The listing builds one solid part. Answer for the finished solid, in the listing's coordinates (mm). Face numbers are marked on the shaded views. A direction names the side the tool comes from. Give positions to 0.01 mm unless a question says otherwise; leave off trailing zeros. Order: outer loops, then holes, each group sorted by start corner. A loop starts at its lowest first (then second) coordinate and runs counter-clockwise, first axis right, second up. Notation, with made-up numbers: (18.25, 68.5) - (56.25, 68.5) arc R20 ccw to (56.25, 99.5) - close; hole circle Ø1 at (-38.5, 11.25). An arc over 180 degrees is marked (long way). Answer in a Markdown table with one row per item.
from build123d import *

# Parameters (mm, degrees)
SKETCH1_W                   = 62.178178995
SKETCH1_H                   = 55.159619557
BOSS_EXTRUDE1_DEPTH         = 3.175
F_1_4_0_25_DIAMETER_HOLE1_D = 6.35
CUT_EXTRUDE6_DEPTH          = 84.179265432
FILLET1_R                   = 8.382
SKETCH7_W                   = 19.05
SKETCH7_H                   = 3.175
BOSS_EXTRUDE2_DEPTH         = 3.175


with BuildPart() as part:
    # Sketch1 → Boss-Extrude1 (new body)
    with BuildSketch(Plane.XY):
        with Locations((-31.089089498, 27.579809779)):
            Rectangle(SKETCH1_W, SKETCH1_H)
    extrude(amount=BOSS_EXTRUDE1_DEPTH)

    # 1/4 (0.25) Diameter Hole1 (through all)
    with Locations(Plane(origin=(0, 0, 0), x_dir=(-1, 0, 0), z_dir=(0, 0, -1))):
        with Locations((42.112178995, 18.542)):
            Hole(F_1_4_0_25_DIAMETER_HOLE1_D / 2)

    # Sketch4 → Cut-Extrude6 (cut, through all)
    with BuildSketch(Plane(origin=(0, 0, 0), x_dir=(-1, 0, 0), z_dir=(0, 0, -1))):
        Polygon((46.938178995, 26.4795), (62.178178995, 0), (62.178178995, 55.159619557), (0, 55.159619557), (0, 0), (24.636978995, 0), (36.778178995, 26.4795), align=None)
    extrude(amount=-CUT_EXTRUDE6_DEPTH, mode=Mode.SUBTRACT)

    # Fillet1
    # the kernel refuses this fillet: 8.382 mm, written as the material it takes off along each edge
    with BuildSketch(Plane(origin=(-46.938178995, 26.4795, -12.117368839), x_dir=(-0.49882253176769886, -0.8667041489463767, 0), z_dir=(0, 0, 1))) as fillet1_piece_1:
        with BuildLine():
            CenterArc((FILLET1_R * 0.578256685216, FILLET1_R), FILLET1_R, 209.922129856, 60.077870144)
            Line((-FILLET1_R * 0.288447463731, FILLET1_R * 0.501177468232), (0, 0))
            Line((0, 0), (FILLET1_R * 0.578256685216, 0))
        make_face()
    extrude(amount=27.409737677, mode=Mode.SUBTRACT)
    with BuildSketch(Plane(origin=(-36.778178995, 26.4795, -13.444588142), x_dir=(0.41678981361521655, -0.9090028884808855, 0), z_dir=(0, 0, 1))) as fillet1_piece_2:
        with BuildLine():
            CenterArc((FILLET1_R * 0.641593325803, -FILLET1_R), FILLET1_R, 90, 65.367919757)
            Line((-FILLET1_R * 0.267409562678, -FILLET1_R * 0.583210186385), (0, 0))
            Line((0, 0), (FILLET1_R * 0.641593325803, 0))
        make_face()
    extrude(amount=30.064176284, mode=Mode.SUBTRACT)

    # Sketch7 → Boss-Extrude2 (add)
    with BuildSketch(Plane(origin=(0, 0, 0), x_dir=(-1, 0, 0), z_dir=(0, 0, -1))):
        with Locations((43.001178995, -1.5875)):
            Rectangle(SKETCH7_W, SKETCH7_H)
    extrude(amount=-BOSS_EXTRUDE2_DEPTH)


solid = part.part
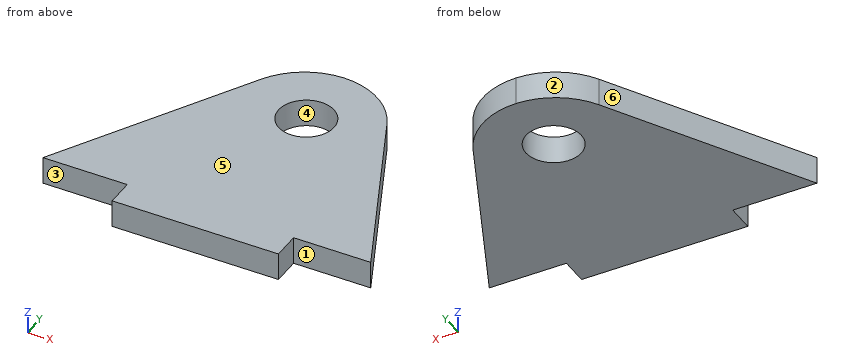
Item 1: Which of the six approach directions +Z, -Z, +X, -X, +Y, -Y give full straight-line access (tool end or side, diameter ignored) to the marked faces 1, 2 and 3?
Answer block:
| item | result |
|---|---|
| face 1 | +Z, -Z, +X, -Y |
| face 2 | +Z, -Z, -X, +Y |
| face 3 | +Z, -Z, -X, -Y |
Item 2: Find section A-A on x = -43.5. Write down the section's boundary in (y, z) (3 decimals), then the cut area to 3 significant figures.
Answer block:
| item | result |
|---|---|
| outline | (-3.175, 0) - (15.686, 0) - (15.686, 3.175) - (-3.175, 3.175) - close; (21.398, 0) - (26.36, 0) - (26.36, 3.175) - (21.398, 3.175) - close |
| area | 75.6 mm² |
Item 3: Determine the mould class of the marked faces 4, 5 and 6 for opening direction X: pulls with the +X half, pulls with the -X half, needs draft (parallel to the pull), parting line crosses it, or undercut.
Answer block:
| item | result |
|---|---|
| face 4 | undercut |
| face 5 | needs draft |
| face 6 | pulls with the -X half |
Item 4: Each of these flat-tipped pins is pushed along its axis until it touches: P1, Ø1.5, axis at y = 7, z = 1.5, coming from the +X side; P2, Ø1, axis at x = -55, z = 2, coming from the -Y side. Where does it stop, or does it pass through?
Answer block:
| item | result |
|---|---|
| P1 | x = -27.5 |
| P2 | y = 0 |
Item 5: Consider line 1 (X direction, y = 17, z = 0.8); line 2 (X direction, y = -1.5, z = 1.5); line 3 (Y direction, x = -41.5, z = 1.1) (3 decimals). Determine where each line is inside the solid, lowest interval first.
Answer block:
| item | result |
|---|---|
| line 1 | -52.39 to -44.89, -39.34 to -32.43 |
| line 2 | -52.53 to -33.48 |
| line 3 | -3.175 to 15.427, 21.657 to 26.454 |
Item 6: Find section C-C on x = -47.5. Write down the section's boundary in (y, z) (3 decimals).
Answer block:
| item | result |
|---|---|
| outline | (-3.175, 0) - (24.501, 0) - (24.501, 3.175) - (-3.175, 3.175) - close |
Item 7: Find section D-D on y = 3.5. Write down the section's boundary in (x, z) (3 decimals).
Answer block:
| item | result |
|---|---|
| outline | (-60.164, 0) - (-26.242, 0) - (-26.242, 3.175) - (-60.164, 3.175) - close |
